The drawing under review shows one solid part. Ordinate dimensions are in mm from its lowest x, y, z. Coordinates: 2 decimals unless noted, no trailing zeros. Loops run counter-clockwise (first coordinate to the right, second up) from the corner with the lowest first, then second, coordinate; pieces in that order, holes last. Notation, with made-up numbers: M 69.25,72.25 L 99.25,72.25 A28 ccw 99.25,106.25 Z; hole C 87,30 d2. An arc over 180 degrees is marked long. Put each result on its own line as item: value.
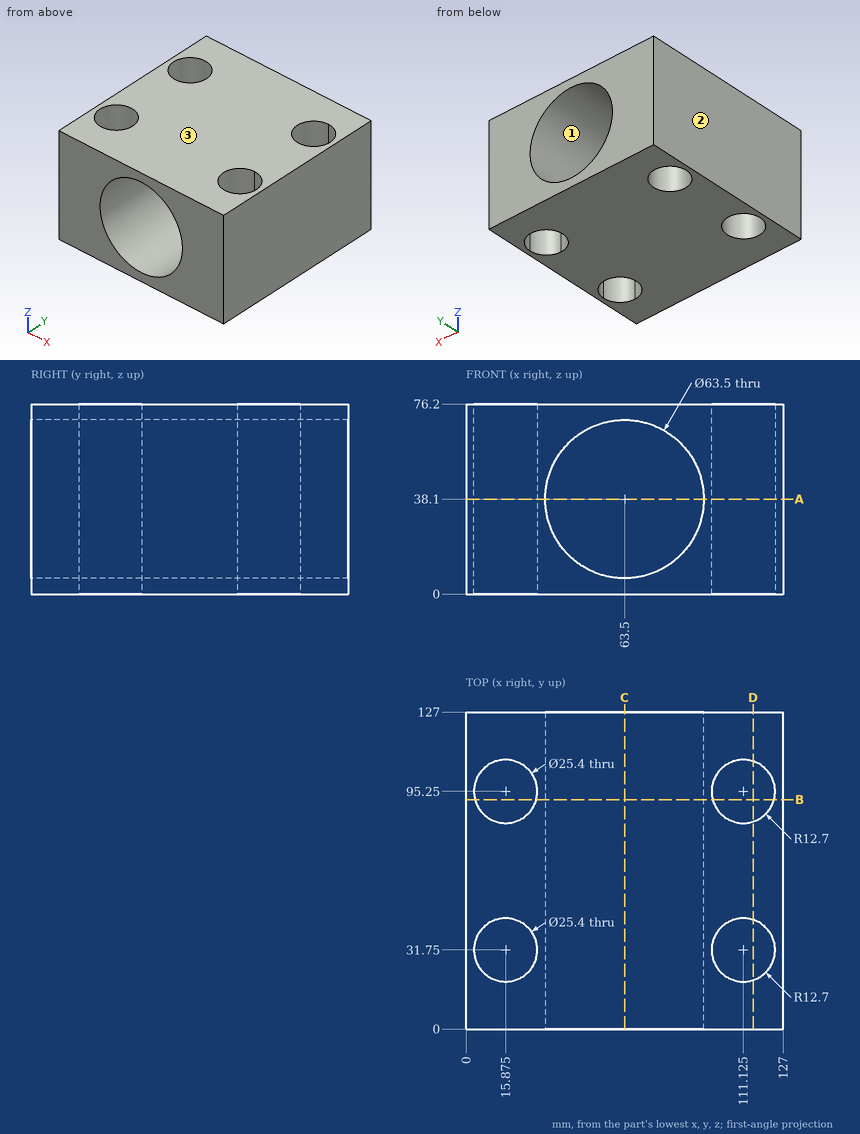
(1) Add section B-B (y = 92). Write out the cut boundary in (x, z).
Determined:
outline: M 0,0 L 3.6,0 L 3.6,76.2 L 0,76.2 Z; M 28.15,0 L 98.85,0 L 98.85,76.2 L 28.15,76.2 Z; M 123.4,0 L 127,0 L 127,76.2 L 123.4,76.2 Z; hole C 63.5,38.1 d63.5
(2) Draft analysis for pull direction X (two halves, no side actions). For the marked faces 1, 2 and 3, state which applies: +X half, -X half, draft (parallel to the pull), parting line (faces both ways), or undercut.
Determined:
face 1: undercut
face 2: -X half
face 3: draft
(3) Add section A-A (z = 38.1). Write out the cut boundary in (x, y) (3 decimals), plus the area to 3 significant figures.
Determined:
outline: M 0,0 L 31.75,0 L 31.75,127 L 0,127 Z; M 95.25,0 L 127,0 L 127,127 L 95.25,127 Z; hole C 15.875,31.75 d25.4; hole C 15.875,95.25 d25.4; hole C 111.125,31.75 d25.4; hole C 111.125,95.25 d25.4
area: 6,040 mm^2
(4) Wall thickness on line 1 along Y through (x, z) = (23, 33.5); line 2 along X through (y, z) = (69, 38); line 3 along X through (y, z) = (31, 26): over which ranges is each line inside the solid? List them lowest first. Write a range as [from, to].
Determined:
line 1: y = [0, 21.24], [42.26, 84.74], [105.76, 127]
line 2: x = [0, 31.75], [95.25, 127]
line 3: x = [0, 3.2], [28.55, 34.15], [92.85, 98.45], [123.8, 127]
(5) Add section C-C (x = 63.5). Write out the cut boundary in (y, z).
Determined:
outline: M 0,0 L 127,0 L 127,6.35 L 0,6.35 Z; M 0,69.85 L 127,69.85 L 127,76.2 L 0,76.2 Z
(6) Add section D-D (x = 115). Write out the cut boundary in (y, z).
Determined:
outline: M 0,0 L 19.66,0 L 19.66,76.2 L 0,76.2 Z; M 43.84,0 L 83.16,0 L 83.16,76.2 L 43.84,76.2 Z; M 107.34,0 L 127,0 L 127,76.2 L 107.34,76.2 Z
